Autodesk Inventor part; units mm, degrees
ref_plane "YZ Plane" through (0, 0, 0) normal (1, 0, 0) x (0, 1, 0)
ref_plane "XZ Plane" through (0, 0, 0) normal (0, 1, 0) x (-1, 0, 0)
ref_plane "XY Plane" through (0, 0, 0) normal (0, 0, 1) x (1, 0, 0)
sketch "Sketch1" plane through (0, 0, 0) normal (0, 0, 1) x (1, 0, 0)
  line L0 (0, 0) -> (25.4, 0)
  line L1 (25.4, 0) -> (25.4, 25.4)
  line L2 (25.4, 25.4) -> (0, 25.4)
  line L3 (0, 25.4) -> (0, 0)
  dimension "d0" = 25.4
  dimension "d1" = 25.4
extrude "Extrusion1" add sketch "Sketch1" along normal blind 88.9
shell "Shell1" thickness 1.5875 removed faces 2 at (8.4667, 16.9333, 0) at (8.4667, 16.9333, 88.9)
properties part number "Frame_FrontConveyorGuideSideSupport"
Check sheet for the modelled part. Datum: model origin and axes. Units: mm. A direction names the side the tool comes from. Give positions to 0.01 mm unless a question says otherwise; leave off trailing zeros. Loops run counter-clockwise (first coordinate to the right, second up) from the corner with the lowest first, then second, coordinate; pieces in that order, holes last. Notation, with made-up numbers: M 70.25,-31.5 L 122.25,-31.5 A21 ccw 122.25,-16.5 Z; hole C 82.5,75 d11. An arc over 180 degrees is marked long. Use a Markdown table: item, result. Add a question column.
Q1. Sectioned sample at C-C, the plane z = 34.5. Record the cut outline in (x, y).
Q2. Tool access check on faces 5 (the flat face through (25.4, 13, 44)), 6 (the flat face through (1.588, 13, 44)). Record the directions out of +Z, -Z, +X, -X, +Y, -Y that give a thin tool (end or side, any length) a straight path to the whole face; none if there is none.
Q3. Mould release check, pull along Y, two halves, no side actions. Record for faces 1 (the flat face through (23.812, 13, 44)), 2 (the flat face through (13, 25.4, 44)), 3 (the flat face through (13, 0, 44)), 4 (the flat face through (13, 23.812, 44)): pulls with the +Y half, pulls with the -Y half, needs draft (parallel to the pull), parting line crosses it, or undercut.
Q4. Sectioned sample at A-A, the plane y = 19.5. Record the cut outline in (x, z), then the cut area to 3 significant figures.
Q5. Scan line: line 1 along Y through (x, z) = (2, 5.5). Record every from-to range of solid material in increasing order. Write a range as [from, to].
Q6. Go/stop test with a flat-tipped pin: pin 1 (12 mm diameter, centred on x = 8.5, y = 11, fed in from +Z). Record where the tip stops, or that it passes through.
Verdict:
| question | item | result |
|---|---|---|
| 1 | outline | M 0,0 L 25.4,0 L 25.4,25.4 L 0,25.4 Z; hole M 1.59,1.59 L 23.81,1.59 L 23.81,23.81 L 1.59,23.81 Z |
| 2 | face 5 | +Z, -Z, +X, +Y, -Y |
| 2 | face 6 | +Z, -Z |
| 3 | face 1 | undercut |
| 3 | face 2 | pulls with the +Y half |
| 3 | face 3 | pulls with the -Y half |
| 3 | face 4 | undercut |
| 4 | outline | M 0,0 L 1.59,0 L 1.59,88.9 L 0,88.9 Z; M 23.81,0 L 25.4,0 L 25.4,88.9 L 23.81,88.9 Z |
| 4 | area | 282 mm^2 |
| 5 | line 1 | [0, 1.59], [23.81, 25.4] |
| 6 | pin 1 | through |
